Part print with two shaded views. Sizes in mm from the minimum x, y, z corner. Coordinates: 2 decimals unless noted, no trailing zeros. Write each loop counter-clockwise with the first axis right and the second up, starting at its lowest first coordinate (ties: lowest second). Pieces come first, ordered by that corner, then holes. Notation, with made-up numbers: (21, 10.25) - (31, 10.25) arc R29 ccw to (31, 41.25) - close; hole circle Ø6 at (14, 21). An arc over 180 degrees is marked (long way). Answer in a Markdown table with one row per item. Add a question column.
Q1. Band-saw the part on B-B (z = 3). List the corners of the cut face in (x, y), and give its area (3 significant figures).
Q2. Drill centre lines: line 1 along Y through (x, z) = (6.75, 2.5); line 2 along X through (y, z) = (1.6, 1.05); line 3 along X through (y, z) = (1.45, 4.45). Where is each one in solid material? Low to high. Write a range as from..to.
Q3. Two-plate mould, pull along Y, no slides. Class the marked faces 1, 2, 3 and 4: +Y half, -Y half, draft (parallel to the pull), parting line (faces both ways), or undercut.
Q4. Pin check, flat tips, straight feed: pin 1 (3 mm diameter, centred on x = 12, y = 1, fed in from +Z); pin 2 (1.8 mm diameter, centred on x = 0.5, z = 2, fed in from -Y); pin 3 (0.5 mm diameter, centred on y = 3, z = 2, fed in from -X). Stop position of each tip, or through.
Q5. Band-saw the part on C-C (x = 13.5). List the corners of the cut face in (y, z), and give its area (3 significant figures).
Q6. Band-saw the part on A-A (y = 3). List the corners of the cut face in (x, z).
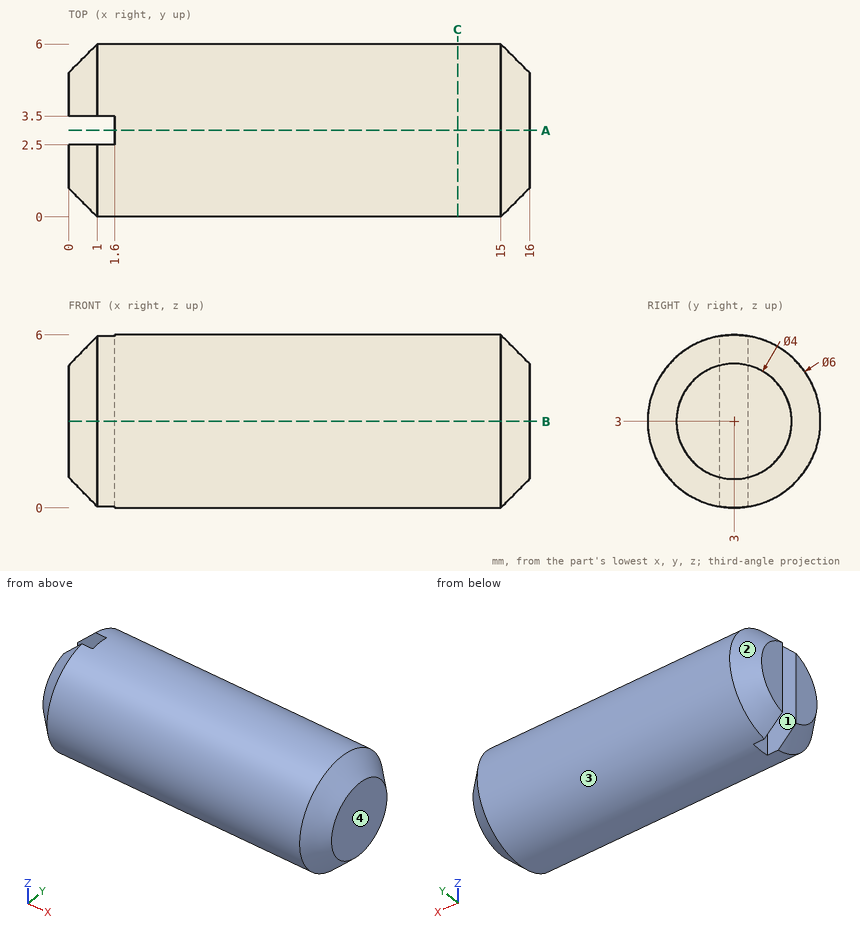
Checked values:
| question | item | result |
|---|---|---|
| 1 | outline | (0, 1) - (1, 0) - (15, 0) - (16, 1) - (16, 5) - (15, 6) - (1, 6) - (0, 5) - (0, 3.5) - (1.6, 3.5) - (1.6, 2.5) - (0, 2.5) - close |
| 1 | area | 92.4 mm² |
| 2 | line 1 | y = 0.04..5.96 |
| 2 | line 2 | x = 0.4..15.6 |
| 2 | line 3 | x = 0.12..15.88 |
| 3 | face 1 | undercut |
| 3 | face 2 | +Y half |
| 3 | face 3 | parting line |
| 3 | face 4 | draft |
| 4 | pin 1 | stops at z = 5.96 |
| 4 | pin 2 | stops at y = 0.01 |
| 4 | pin 3 | stops at x = 1.6 |
| 5 | outline | circle Ø6 at (3, 3) |
| 5 | area | 28.3 mm² |
| 6 | outline | (1.6, 0) - (15, 0) - (16, 1) - (16, 5) - (15, 6) - (1.6, 6) - close |
